Verification items for the finished model (mm, model axes). Face numbers are marked on the shaded views. A direction names the side the tool comes from. Round coordinates to 2 decimals unless told otherwise and drop trailing zeros. Order: outer loops, then holes, each group sorted by start corner. A loop starts at its lowest first (then second) coordinate and runs counter-clockwise, first axis right, second up. Notation, with made-up numbers: M 61.5,62.5 L 82.5,62.5 A20 ccw 82.5,71.5 Z; hole C 38,4 d1. An arc over 180 degrees is marked long. Answer as a JSON object with one key per item and string values. Group by question number.
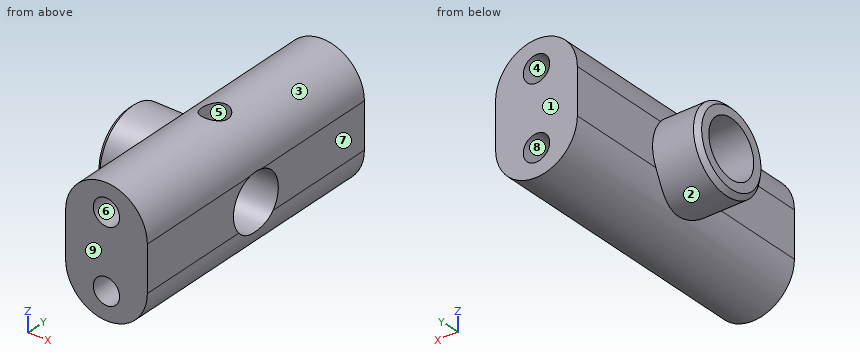
Autodesk Inventor part; units mm, degrees
ref_plane "Work Plane9" through (0, 0, -0.5) normal (0, 0, 1) x (1, 0, 0)
ref_plane "YZ Plane" through (0, 0, 0) normal (1, 0, 0) x (0, 1, 0)
ref_plane "XZ Plane" through (0, 0, 0) normal (0, 1, 0) x (-1, 0, 0)
sketch "Sketch2" plane through (0, 0, 0) normal (0, 1, 0) x (-1, 0, 0)
  line L0 (-4.5, -10) -> (-4.5, -5)
  line L1 (4.5, -10) -> (4.5, -5)
  arc A0 (4.5, -5) -> (-4.5, -5) centre (0, -5) ccw
  arc A1 (-4.5, -10) -> (4.5, -10) centre (0, -10) ccw
  point P0 (0, 0)
  point P1 (0.9888, -13.1808)
  dimension "d75" = 5
  dimension "d76" = 5
extrude "Extrusion1" add sketch "Sketch2" along normal blind 30
sketch "Sketch14" plane through (-4.5, 0, -10) normal (-1, 0, 0) x (0, 0, 1)
  line L0 (-4.5, 0) -> (-4.5, 30)
  line L1 (-4.5, 0) -> (-4.5, 15)
  line L2 (-4.5, 15) -> (2, 15)
  circle A0 centre (2, 15) radius 3.1
  circle A1 centre (2, 15) radius 4.6
  point P0 (10, 0)
  point P1 (-11.5, 30)
  dimension "d80" = 15
  dimension "d81" = 6.5
  dimension "d82" = 6.2
  dimension "d83" = 9.2
extrude "Extrusion13" add sketch "Sketch14" along normal blind 5 and the other way blind 5
chamfer "Chamfer4" distance 0.5 angle 45 1 edges at (-9.5, 15, -12.6)
sketch "Sketch15" plane through (-4.5, 15, -8) normal (-1, 0, 0) x (0, 0, 1)
  circle A0 centre (0, 0) radius 3.1
  point P0 (8, -15)
extrude "Extrusion14" cut sketch "Sketch15" against normal through all
sketch "Sketch18" plane through (0, 30, 0) normal (0, 1, 0) x (1, 0, 0)
  arc A0 (4.5, 10) -> (-4.5, 10) centre (0, 10) ccw
  line L0 (0, 14.5) -> (0, 11.5)
  circle A1 centre (0, 11.5) radius 1.45
  arc A2 (-4.5, 5) -> (4.5, 5) centre (0, 5) ccw
  line L1 (0, 0.5) -> (0, 3.5)
  circle A3 centre (0, 3.5) radius 1.45
  point P0 (0, 0)
  dimension "d103" = 3
  dimension "d104" = 2.9
  dimension "d105" = 3
  dimension "d106" = 2.9
extrude "Extrusion17" cut sketch "Sketch18" against normal blind 10
sketch "Sketch19" plane through (0, 0, 0) normal (0, -1, 0) x (1, 0, 0)
  line L0 (4.5, -10) -> (4.5, -5)
  arc A0 (4.5, -5) -> (-4.5, -5) centre (0, -5) ccw
  line L1 (-4.5, -5) -> (-4.5, -10)
  arc A1 (-4.5, -10) -> (4.5, -10) centre (0, -10) ccw
  circle A2 centre (0, -11.5) radius 1.45
  circle A3 centre (0, -3.5) radius 1.45
extrude "Extrusion18" cut sketch "Sketch19" against normal blind 10 contours A2 | A3
ref_plane "Work Plane9" through (0, 0, -0.5) normal (0, 0, 1) x (1, 0, 0)
sketch "Sketch20" plane through (0, 0, 0) normal (0, 0, 1) x (1, 0, 0)
  circle A0 centre (0, 15) radius 1.45
  point P0 (0, 0)
  dimension "d115" = 2.9
extrude "Extrusion19" cut sketch "Sketch20" against normal up to next
thread "Thread1"
properties part number "Front mount" material "ABS Plastic"
Q1. Cross-section at B-B, the plane y = 15. Record the cut outline in (x, z).
Q2. Gauge pin test, flat ends, axial feed: pin 1 Ø5.5 at (y, z) = (27, -7) entering from -X; pin 2 Ø2.5 at (x, z) = (0, -3.5) entering from +Y; pin 3 Ø1 at (y, z) = (13, -2.5) entering from -X. Record the tip position at first contact, or that the pin passes through.
Q3. Cross-section at C-C, the plane x = 0. Record the cut outline in (y, z), then the cut area to 3 significant figures.
Q4. Thickness scan on line 1 (Z direction, x = 0, y = 24); line 2 (Y direction, x = 0, z = -1.7); line 3 (Y direction, x = -3, z = -8). Record the ranges inside material, lowest first. Write a range as from..to.
Q5. Tool access check on the marked faces 5, 6, 7, 8 and 9. Record the directions out of +Z, -Z, +X, -X, +Y, -Y that give a thin tool (end or side, any length) a straight path to the whole face; none if there is none.
Q6. Cross-section at A-A, the plane z = -8. Record the cut outline in (x, y), then the cut area to 3 significant figures.
Q7. Cross-section at D-D, the plane z = -3. Record the cut outline in (x, y), then the cut area to 3 significant figures.
Q8. Release check for a two-part mould opening along Z. For the marked faces 1, 2, 3 and 4 record: released by +Z, released by -Z, zero draft, split by the parting line, or undercut.
Conclusion:
{
 "1": {"outline": "M -9.5,-12.1 L -9,-12.6 L -3.67,-12.6 A4.5 ccw 4.36,-11.1 L -9.5,-11.1 Z; M -9.5,-4.9 L -1.45,-4.9 L -1.45,-0.74 A4.5 ccw -4.21,-3.4 L -9,-3.4 L -9.5,-3.9 Z; M 1.45,-4.9 L 4.5,-4.9 A4.5 ccw 1.45,-0.74 Z"},
 "2": {"pin 1": "x = -4.5", "pin 2": "y = 20", "pin 3": "x = -4.03"},
 "3": {"outline": "M 0,-14.5 L 30,-14.5 L 30,-12.95 L 20,-12.95 L 20,-10.05 L 30,-10.05 L 30,-4.95 L 20,-4.95 L 20,-2.05 L 30,-2.05 L 30,-0.5 L 16.45,-0.5 L 16.45,-5.26 A3.1 cw long 13.55,-5.26 L 13.55,-0.5 L 0,-0.5 L 0,-2.05 L 10,-2.05 L 10,-4.95 L 0,-4.95 L 0,-10.05 L 10,-10.05 L 10,-12.95 L 0,-12.95 Z", "area": "261 mm2"},
 "4": {"line 1": "-14.5..-12.95, -10.05..-4.95, -2.05..-0.5", "line 2": "0..13.55, 16.45..30", "line 3": "0..11.9, 18.1..30"},
 "5": {"face 5": "+Z", "face 6": "-Y", "face 7": "+Z, -Z, +X, +Y, -Y", "face 8": "+Y", "face 9": "+Z, -Z, +X, -X, -Y"},
 "6": {"outline": "M -9.5,10.9 L -9,10.4 L -4.5,10.4 L -4.5,0 L 4.5,0 L 4.5,11.9 L -9.5,11.9 Z; M -9.5,18.1 L 4.5,18.1 L 4.5,30 L -4.5,30 L -4.5,19.6 L -9,19.6 L -9.5,19.1 Z", "area": "229 mm2"},
 "7": {"outline": "M -4.03,0 L -1.36,0 L -1.36,10 L 1.36,10 L 1.36,0 L 4.03,0 L 4.03,30 L 1.36,30 L 1.36,20 L -1.36,20 L -1.36,30 L -4.03,30 Z; hole C 0,15 d2.9", "area": "181 mm2"},
 "8": {"face 1": "zero draft", "face 2": "split by the parting line", "face 3": "released by +Z", "face 4": "undercut"}
}
